from build123d import *

# Parameters (mm, degrees)
SKETCH039_R     = 30.3
SKETCH039_R_2   = 23.7
PAD008_DEPTH    = 5
SKETCH040_R     = 2.6
POCKET011_DEPTH = 4.2
SKETCH041_R     = 25
SKETCH041_R_2   = 23.7
PAD009_DEPTH    = 30
CHAMFER_SIZE2   = 5
CHAMFER_SIZE    = 4.999
SKETCH043_R     = 26.3
SKETCH043_R_2   = 25
PAD010_DEPTH    = 7.5
CHAMFER001_SIZE = 1.29
CHAMFER002_SIZE = 2.59


with BuildPart() as part:
    # Sketch039 → Pad008 (new body)
    with BuildSketch(Plane(origin=(0, 0, 0), x_dir=(-0.3826834324, 0.9238795325, 0), z_dir=(0, 0, 1))):
        with Locations((0, -80)):
            Circle(SKETCH039_R)
        with Locations((0, -80)):
            Circle(SKETCH039_R_2, mode=Mode.SUBTRACT)
    extrude(amount=PAD008_DEPTH)

    # Sketch040 → Pocket011 (cut)
    with BuildSketch(Plane(origin=(0, 0, 0), x_dir=(-0.3826834324, 0.9238795325, 0), z_dir=(0, 0, 1))):
        with Locations((0, -53)):
            Circle(SKETCH040_R)
        with Locations((-23.3826859022, -66.5)):
            Circle(SKETCH040_R)
        with Locations((-23.3826859022, -93.5)):
            Circle(SKETCH040_R)
        with Locations((0, -107)):
            Circle(SKETCH040_R)
        with Locations((23.3826859022, -93.5)):
            Circle(SKETCH040_R)
        with Locations((23.3826859022, -66.5)):
            Circle(SKETCH040_R)
        with Locations((-13.5, -56.6173140978)):
            Circle(SKETCH040_R)
        with Locations((-27, -80)):
            Circle(SKETCH040_R)
        with Locations((-13.5, -103.3826859022)):
            Circle(SKETCH040_R)
        with Locations((13.5, -103.3826859022)):
            Circle(SKETCH040_R)
        with Locations((27, -80)):
            Circle(SKETCH040_R)
        with Locations((13.5, -56.6173140978)):
            Circle(SKETCH040_R)
    extrude(amount=POCKET011_DEPTH, mode=Mode.SUBTRACT)

    # Sketch041 → Pad009 (join)
    with BuildSketch(Plane(origin=(0, 0, 5), x_dir=(-0.3826834324, 0.9238795325, 0), z_dir=(0, 0, 1))):
        with Locations((0, -80)):
            Circle(SKETCH041_R)
        with Locations((0, -80)):
            Circle(SKETCH041_R_2, mode=Mode.SUBTRACT)
    extrude(amount=PAD009_DEPTH)

    # Chamfer
    chamfer_edges = [part.edges().sort_by_distance(p)[0] for p in [
        (83.477448, 7.517686, 5),
    ]]
    chamfer_side = part.faces().sort_by_distance((85.177706, 3.412902, 5))[0]
    chamfer(chamfer_edges, length=CHAMFER_SIZE, length2=CHAMFER_SIZE2, reference=chamfer_side)

    # Sketch043 → Pad010 (join)
    with BuildSketch(Plane(origin=(0, 0, 27.5), x_dir=(-0.3826834324, 0.9238795325, 0), z_dir=(0, 0, 1))):
        with Locations((0, -80)):
            Circle(SKETCH043_R)
        with Locations((0, -80)):
            Circle(SKETCH043_R_2, mode=Mode.SUBTRACT)
    extrude(amount=PAD010_DEPTH)

    # Chamfer001
    chamfer001_edges = [part.edges().sort_by_distance(p)[0] for p in [
        (83.974937, 6.316643, 27.5),
    ]]
    chamfer(chamfer001_edges, length=CHAMFER001_SIZE)

    # Chamfer002
    chamfer002_edges = [part.edges().sort_by_distance(p)[0] for p in [
        (82.97996, 8.71873, 35),
    ]]
    chamfer(chamfer002_edges, length=CHAMFER002_SIZE)


with BuildPart() as part_1:
    # Body006 placement: moved
    add(part.part.moved(Location((0, 0, 100))))


solid = part_1.part
Part model, mm, in its own coordinate system. A direction names the side the tool comes from. Give positions to 0.01 mm unless a question says otherwise; leave off trailing zeros. Loops run counter-clockwise (first coordinate to the right, second up) from the corner with the lowest first, then second, coordinate; pieces in that order, holes last.
(1) Band-saw the part on B-B (z = 107.5). Write the cut outline in (x, y), and give its area (3 significant figures).
Return value:
outline: circle Ø55 at (73.91, 30.61); hole circle Ø47.4 at (73.91, 30.61)
area: 611 mm2
(2) Band-saw the part on A-A (z = 103). Count the separate pieces of the cut face and the enclosed holes in it, and give its area (3 significant figures).
Return value:
separate pieces: 1
enclosed holes: 13
area: 865 mm2
(3) Pin check, flat tips, straight feed: pin 1 (1.6 mm diameter, centred on x = 98, y = 40.5, fed in from -Z); pin 2 (8 mm diameter, centred on x = 50.5, z = 129.5, fed in from +Y); pin 3 (12 mm diameter, centred on x = 81.5, y = 49, fed in from +Z). Stop position of each tip, or through.
Return value:
pin 1: stops at z = 104.2
pin 2: stops at y = 48.36
pin 3: stops at z = 134.6
(4) Band-saw the part on C-C (z = 113). Write the cut outline in (x, y).
Return value:
outline: circle Ø50 at (73.91, 30.61); hole circle Ø47.4 at (73.91, 30.61)
(5) 3-axis set-ups, long thin cutter, end or side, ignore diameter. For faces 4 (the cylindrical face through (52.255, 18.122, 118.628)), 5 (the flat face through (90, 52, 104.2)), 6 (the cylindrical face through (58.683, 48.775, 115.978)): which of +Z, -Z, +X, -X, +Y, -Y reach the whole face in a straight line?
Return value:
face 4: none
face 5: -Z
face 6: +Z, -Z
(6) Drill centre lines: line 1 along X through (y, z) = (57, 102.5); line 2 along Y through (x, z) = (57.5, 103.5); line 3 along Y through (x, z) = (52.5, 113). Where is each one in solid material? Low to high.
Return value:
line 1: x = 59.01 to 61.41, 65.74 to 74.86, 80.01 to 88.81
line 2: y = 5.14 to 6.59, 11.79 to 13.52, 47.71 to 56.09
line 3: y = 17.71 to 20.45, 40.78 to 43.52
(7) Pull direction Y, two halves, no side cores. Call faces 1 (the cylindrical face through (44.073, 35.887, 102.465)), 2 (the cylindrical face through (67.826, 4.298, 102.071)), 3 (the cylindrical face through (76.544, 54.941, 102.071)): pulls with the +Y half, pulls with the -Y half, needs draft (parallel to the pull), parting line crosses it, or undercut.
Return value:
face 1: parting line crosses it
face 2: undercut
face 3: undercut
